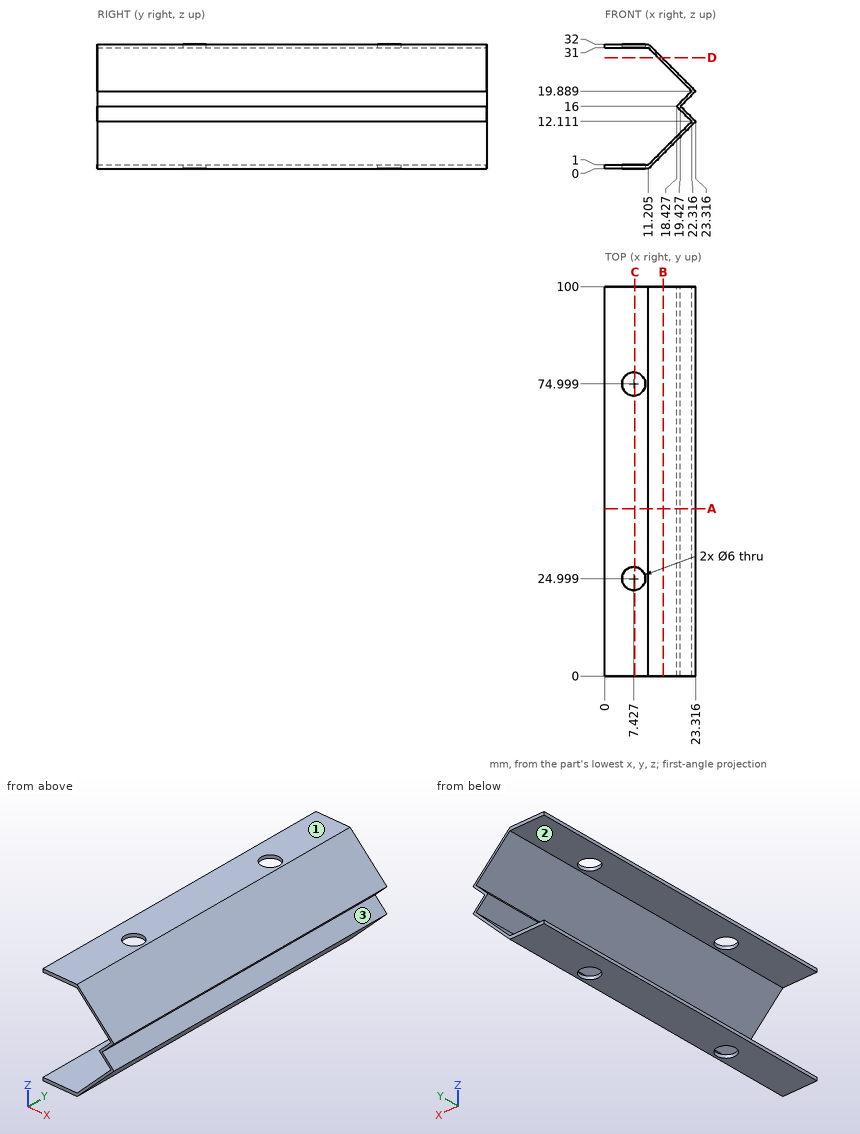
For this review, use the dimensioned drawing (mm, ordinates from the lowest corner) and the shaded views. A direction names the side the tool comes from. Round coordinates to 2 decimals unless told otherwise and drop trailing zeros. Order: outer loops, then holes, each group sorted by start corner. A loop starts at its lowest first (then second) coordinate and runs counter-clockwise, first axis right, second up. Notation, with made-up numbers: (-40, -23.5) - (3, -23.5) arc R9 ccw to (3, -7.5) - close; hole circle Ø6 at (23, -37.5). An arc over 180 degrees is marked (long way). Use one line per item in the form item = value.
Q1. Tool access review of the marked faces 1, 2 and 3: name each direction out of +Z, -Z, +X, -X, +Y, -Y from which nothing blocks a thin tool from reaching the whole face with its end or side.
Response values:
face_1 = +Z, +X, -X, +Y, -Y
face_2 = -X, +Y, -Y
face_3 = +X, +Y, -Y
Q2. Add section D-D on z = 28.5. Give the boundary of the cut face in (x, y) (1 decimal).
Response values:
outline = (13.7, 0) - (14.7, 0) - (14.7, 100) - (13.7, 100) - close
Q3. To check wall thickness, follow line 1 (Z direction, x = 6.5, y = 14.5); line 2 (Z direction, x = 19.25, y = 52) (1 decimal); line 3 (Z direction, x = 21.25, y = 43) (1 decimal). State the ranges of each line that lie inside material, in increasing order.
Response values:
line_1 = 0 to 1, 31 to 32
line_2 = 8 to 9, 15.2 to 16.8, 23 to 24
line_3 = 10 to 11, 13.2 to 14.2, 17.8 to 18.8, 21 to 22
Q4. Add section B-B on x = 15. Give the boundary of the cut face in (y, z) (1 decimal).
Response values:
outline = (0, 3.8) - (100, 3.8) - (100, 4.8) - (0, 4.8) - close; (0, 27.2) - (100, 27.2) - (100, 28.2) - (0, 28.2) - close
Q5. Add section A-A on y = 43. Give the boundary of the cut face in (x, z) (1 decimal).
Response values:
outline = (0, 0) - (11.2, 0) - (23.3, 12.1) - (19.4, 16) - (23.3, 19.9) - (11.2, 32) - (0, 32) - (0, 31) - (11.2, 31) - (22.3, 19.9) - (18.4, 16) - (22.3, 12.1) - (11.2, 1) - (0, 1) - close
Q6. Clearance check with flat-ended pins moving along their axes: P1, Ø1, axis at y = 61, z = 16, coming from the +X side; P2, Ø12, axis at y = 12.5, z = 28.5, coming from the +X side (1 decimal); P3, Ø5, axis at y = 62, z = 12, coming from the +X side. State where each tip first meets the part, or that it passes through.
Response values:
P1 = 19.93
P2 = 20.7
P3 = 23.32
Q7. Add section C-C on x = 7.75. Give the boundary of the cut face in (y, z).
Response values:
outline = (0, 0) - (22.02, 0) - (22.02, 1) - (0, 1) - close; (0, 31) - (22.02, 31) - (22.02, 32) - (0, 32) - close; (27.98, 0) - (72.02, 0) - (72.02, 1) - (27.98, 1) - close; (27.98, 31) - (72.02, 31) - (72.02, 32) - (27.98, 32) - close; (77.98, 0) - (100, 0) - (100, 1) - (77.98, 1) - close; (77.98, 31) - (100, 31) - (100, 32) - (77.98, 32) - close
